Input: part model. Units: mm. Frame: model coordinates. A direction names the side the tool comes from. Round coordinates to 2 decimals unless told otherwise and drop trailing zeros. Loops run counter-clockwise (first coordinate to the right, second up) from the corner with the lowest first, then second, coordinate; pieces in that order, holes last.
1) Section B-B, the plane y = 8.5. Return loops of the section in (x, z), and give its area (3 significant figures).
2) First-contact query: pin 1 (1.6 mm diameter, centred on x = 1.5, y = 67.5, fed in from -Z); pin 2 (6 mm diameter, centred on x = 13.5, y = 22, fed in from -Z); pin 3 (10 mm diameter, centred on x = 5, z = 21.5, fed in from +Y); pin 4 (8.5 mm diameter, centred on y = 75, z = 47, fed in from -X). Flat tips, straight axial feed; report the tip coordinate or a pass-through.
3) Section A-A, the plane z = 7.5. Return loops of the section in (x, y), and give its area (3 significant figures).
4) Section D-D, the plane x = 16. Return loops of the section in (y, z).
5) Access query for faces 1 (the face through (8, 4, 4)), 2 (the face through (1, 66, 38)), 3 (the face through (8.93, 2.03, 65.77)). Directions: +Z, -Z, +X, -X, +Y, -Y. A direction counts if a zero-diameter tool reaches every point of the face in a straight line with its end or side. Return the directions, or none.
6) Draft query along Y for faces 4 (the face through (10, 44, 17)), 5 (the face through (20, 44, 43)), 6 (the face through (1.945, 66, 53)). Return one class per face: pulls with the +Y half, pulls with the -Y half, needs draft (parallel to the pull), parting line crosses it, or undercut.
7) Section C-C, the plane x = 8.5. Return loops of the section in (y, z), and give its area (3 significant figures).
8) Ray query, line 1 along Z through (x, y) = (8.5, 2.7); line 2 along Y through (x, z) = (4.25, 7.5); line 3 along Y through (x, z) = (14.75, 66). Return the intervals inside material, ascending.
from build123d import *

# Parameters (mm, degrees)
SKETCH004_W  = 43
SKETCH004_H  = 29
PAD004_DEPTH = 2
SKETCH003_W  = 17
SKETCH003_H  = 37
PAD003_DEPTH = 70
SKETCH001_W  = 41
SKETCH001_H  = 40
PAD001_DEPTH = 20
SKETCH002_W  = 46
SKETCH002_H  = 35
PAD002_DEPTH = 20
SKETCH_W     = 90
SKETCH_H     = 70
PAD_DEPTH    = 20
SKETCH005_R  = 3.3
HOLE_DEPTH   = 4.001


with BuildPart() as body004:
    # Sketch004 (on Face1 of CopyPad003) → Pad004 (new body)
    with BuildSketch(Plane(origin=(-0.05496, 0, 0), x_dir=(0, -1, 0), z_dir=(-1, 0, 0))):
        with Locations((-65.5, 52.5)):
            Rectangle(SKETCH004_W, SKETCH004_H)
    extrude(amount=-PAD004_DEPTH)


with BuildPart() as body003:
    # Sketch003 (on Face1 of CopyPad002) → Pad003 (new body)
    with BuildSketch(Plane(origin=(0, 0, 0), x_dir=(1, 0, 0), z_dir=(0, 0, -1))):
        with Locations((8.44504, -22.5)):
            Rectangle(SKETCH003_W, SKETCH003_H)
    extrude(amount=-PAD003_DEPTH)


with BuildPart() as body001:
    # Sketch001 (on Face1 of CopyPad) → Pad001 (new body)
    with BuildSketch(Plane(origin=(0, 0, 0), x_dir=(0, -1, 0), z_dir=(-1, 0, 0))):
        with Locations((-20.5, 35)):
            Rectangle(SKETCH001_W, SKETCH001_H)
    extrude(amount=-PAD001_DEPTH)


with BuildPart() as body002:
    # Sketch002 (on Face1 of CopyPad001) → Pad002 (new body)
    with BuildSketch(Plane(origin=(0, 0, 0), x_dir=(0, -1, 0), z_dir=(-1, 0, 0))):
        with Locations((-67, 17.5)):
            Rectangle(SKETCH002_W, SKETCH002_H)
    extrude(amount=-PAD002_DEPTH)


with BuildPart() as body:
    # Sketch → Pad (new body)
    with BuildSketch(Plane.YZ):
        with Locations((45, 35)):
            Rectangle(SKETCH_W, SKETCH_H)
    extrude(amount=PAD_DEPTH)

    # Boolean: cut Body004, Body003, Body001, Body002
    add(body004.part, mode=Mode.SUBTRACT)
    add(body003.part, mode=Mode.SUBTRACT)
    add(body001.part, mode=Mode.SUBTRACT)
    add(body002.part, mode=Mode.SUBTRACT)

    # Sketch005 (on Face24 of Boolean) → Hole (cut, through all)
    with BuildSketch(Plane(origin=(0, 4, 0), x_dir=(-1, 0, 0), z_dir=(0, 1, 0))):
        with Locations((-8.5, 7.5)):
            Circle(SKETCH005_R)
        with Locations((-8.5, 62.5)):
            Circle(SKETCH005_R)
    extrude(amount=-HOLE_DEPTH, mode=Mode.SUBTRACT)


solid = body.part
Final values:
1. outline: (16.95, 0) - (20, 0) - (20, 15) - (16.95, 15) - close; (16.95, 55) - (20, 55) - (20, 70) - (16.95, 70) - close
1. area: 91.6 mm2
2. pin 1: stops at z = 35
2. pin 2: passes through
2. pin 3: stops at y = 44
2. pin 4: stops at x = 1.95
3. outline: (0, 0) - (5.2, 0) - (5.2, 4) - (0, 4) - close; (0, 41) - (16.95, 41) - (16.95, 4) - (11.8, 4) - (11.8, 0) - (20, 0) - (20, 44) - (0, 44) - close
3. area: 227 mm2
4. outline: (0, 0) - (4, 0) - (4, 15) - (0, 15) - close; (0, 55) - (4, 55) - (4, 70) - (0, 70) - close; (41, 0) - (44, 0) - (44, 35) - (90, 35) - (90, 70) - (41, 70) - close
5. face 1: +Z, -Z, -X
5. face 2: -X
5. face 3: -Y
6. face 4: pulls with the +Y half
6. face 5: needs draft
6. face 6: undercut
7. outline: (0, 0) - (4, 0) - (4, 4.2) - (0, 4.2) - close; (0, 10.8) - (4, 10.8) - (4, 15) - (0, 15) - close; (0, 55) - (4, 55) - (4, 59.2) - (0, 59.2) - close; (0, 65.8) - (4, 65.8) - (4, 70) - (0, 70) - close; (41, 0) - (44, 0) - (44, 35) - (90, 35) - (90, 70) - (41, 70) - close
7. area: 1,890 mm2
8. line 1: z = 0 to 4.2, 10.8 to 15, 55 to 59.2, 65.8 to 70
8. line 2: y = 0 to 4, 41 to 44
8. line 3: y = 0 to 4, 41 to 90
